Build history of the part. All positions in model axes, mm. A direction names the side the tool comes from. Round coordinates to 2 decimals unless told otherwise and drop trailing zeros. Order: outer loops, then holes, each group sorted by start corner. A loop starts at its lowest first (then second) coordinate and runs counter-clockwise, first axis right, second up. Notation, with made-up numbers: (-12, 48) -> (-1, 48) arc R9 ccw to (-1, 65) -> close; hole circle Ø6 at (-24, -16.75). An arc over 180 degrees is marked (long way). Use a Markdown table: item, result. Add a question column.
Item 1: Probe L1, parallel to X at y = -18, z = 2; L2, parallel to Z at x = 1, y = -13; L3, parallel to Y at x = 11, z = -1. List the from-to ranges inside material, lowest first.
Item 2: Pin check, flat tips, straight feed: pin 1 (3.5 mm diameter, centred on y = -18, z = 3, fed in from +X); pin 2 (0.6 mm diameter, centred on x = 10.5, z = 0.5, fed in from -Y); pin 3 (3 mm diameter, centred on x = -14, y = -6.5, fed in from +Z). Stop position of each tip, or through.
Item 3: Slice it at C-C, the plane y = -4. Give the cut face in (x, z), plus the area to 3 significant figures.
Item 4: Two-plate mould, pull along X, no slides. Class faces 1 (the face through (13, -8, 1.778)), 2 (the face through (0, -15, 1.778)), 3 (the face through (-14.553, -13.712, 0.025)): released by +X, released by -X, zero draft, split by the parting line, or undercut.
Item 5: Slice it at B-B, the plane z = 0.75. Give the cut face in (x, y).
Item 6: Slice it at D-D, the plane x = -2. Give the cut face in (y, z).
Item 7: Slice it at A-A, the plane z = 3. Give the cut face in (x, y), plus the area to 3 significant figures.
Item 8: 3-axis set-ups, long thin cutter, end or side, ignore diameter. For faces 4 (the face through (6.477, -15, 3)), 5 (the face through (10, -15.24, 0)), 6 (the face through (-10, -15.24, 0)), 7 (the face through (-13, -8, 1.778)): which of +Z, -Z, +X, -X, +Y, -Y reach the whole face in a straight line?
from build123d import *

# Parameters (mm, degrees)
F0_W     = 3.175
F0_H     = 3.048
F1_DEPTH = 30.48
F0_W_2   = 6.35
F0_H_2   = 3.556
F2_DEPTH = 15.24
F3_DEPTH = 15.24
F4_R     = 5.08


with BuildPart() as f1:
    # F0 (on Front) → F1 (new body)
    with BuildSketch(Plane.XZ):
        Polygon((9.652, -1.778), (9.652, 1.778), (6.477, 1.778), (-6.477, 1.778), (-9.652, 1.778), (-9.652, -1.778), align=None)
        with Locations((8.0645, 3.302)):
            Rectangle(F0_W, F0_H)
        with Locations((-8.0645, 3.302)):
            Rectangle(F0_W, F0_H)
    extrude(amount=F1_DEPTH)

    # F0 (on Front) → F2 (join)
    with BuildSketch(Plane.XZ):
        with Locations((12.827, 0)):
            Rectangle(F0_W_2, F0_H_2)
    extrude(amount=F2_DEPTH)

    # F0 (on Front) → F3 (join)
    with BuildSketch(Plane.XZ):
        with Locations((-12.827, 0)):
            Rectangle(F0_W_2, F0_H_2)
    extrude(amount=F3_DEPTH)

    # F4
    f4_edges = [f1.edges().sort_by_distance(p)[0] for p in [
        (-16.002, -15.24, 0),
        (16.002, -15.24, 0),
    ]]
    fillet(f4_edges, radius=F4_R)


solid = f1.part
Check sheet entries:
| question | item | result |
|---|---|---|
| 1 | L1 | -9.65 to -6.48, 6.48 to 9.65 |
| 1 | L2 | -1.78 to 1.78 |
| 1 | L3 | -15.24 to 0 |
| 2 | pin 1 | x = 9.65 |
| 2 | pin 2 | y = -15.24 |
| 2 | pin 3 | z = 1.78 |
| 3 | outline | (-16, -1.78) -> (16, -1.78) -> (16, 1.78) -> (9.65, 1.78) -> (9.65, 4.83) -> (6.48, 4.83) -> (6.48, 1.78) -> (-6.48, 1.78) -> (-6.48, 4.83) -> (-9.65, 4.83) -> (-9.65, 1.78) -> (-16, 1.78) -> close |
| 3 | area | 133 mm2 |
| 4 | face 1 | zero draft |
| 4 | face 2 | undercut |
| 4 | face 3 | released by -X |
| 5 | outline | (-16, -10.16) arc R5.08 ccw to (-10.92, -15.24) -> (-9.65, -15.24) -> (-9.65, -30.48) -> (9.65, -30.48) -> (9.65, -15.24) -> (10.92, -15.24) arc R5.08 ccw to (16, -10.16) -> (16, 0) -> (-16, 0) -> close |
| 6 | outline | (-30.48, -1.78) -> (0, -1.78) -> (0, 1.78) -> (-30.48, 1.78) -> close |
| 7 | outline | (-9.65, -30.48) -> (-6.48, -30.48) -> (-6.48, 0) -> (-9.65, 0) -> close; (6.48, -30.48) -> (9.65, -30.48) -> (9.65, 0) -> (6.48, 0) -> close |
| 7 | area | 194 mm2 |
| 8 | face 4 | +Z, +Y, -Y |
| 8 | face 5 | +Z, -Z, +X, -Y |
| 8 | face 6 | +Z, -Z, -X, -Y |
| 8 | face 7 | +Z, -X, +Y, -Y |
